from build123d import *

# Parameters (mm, degrees)
F0_W          = 1700
F0_H          = 290
F1_DEPTH      = 30
F2_W          = 30
F2_H          = 30
F3_DEPTH      = 600
F4_W          = 290
F4_H          = 30
F5_DEPTH      = 850
F5_DEPTH_BACK = 850


with BuildPart() as f1:
    # F0 (on Top) → F1 (new body)
    with BuildSketch(Plane.XY):
        Rectangle(F0_W, F0_H)
    extrude(amount=F1_DEPTH)

    # F2 (on face) → F3 (join)
    with BuildSketch(Plane(origin=(0, 0, 0), x_dir=(1, 0, 0), z_dir=(0, 0, -1))):
        with Locations((-835, 130)):
            Rectangle(F2_W, F2_H)
        with Locations((835, 130)):
            Rectangle(F2_W, F2_H)
        with Locations((835, -130)):
            Rectangle(F2_W, F2_H)
        with Locations((-835, -130)):
            Rectangle(F2_W, F2_H)
    extrude(amount=F3_DEPTH)

    # F4 (on Right) → F5 (join, two sides)
    with BuildSketch(Plane.YZ) as f5_sk:
        with Locations((0, -315)):
            Rectangle(F4_W, F4_H)
    extrude(amount=F5_DEPTH)
    extrude(f5_sk.sketch, amount=-F5_DEPTH_BACK)


solid = f1.part
Work out the finished part from the listing and answer in its coordinate system (mm). A direction names the side the tool comes from. Coordinates: 2 decimals unless noted, no trailing zeros. Write each loop counter-clockwise with the first axis right and the second up, starting at its lowest first coordinate (ties: lowest second). Pieces come first, ordered by that corner, then holes. Notation, with made-up numbers: M 22,-1 L 42,-1 A24 cw 42,33 Z; hole C 83.5,81.25 d8. An arc over 180 degrees is marked long. Use one line per item in the form item = value. Start each with the question number.
1. This flat-tipped pin is pushed along its axis until it touches: P1, Ø2, axis at x = -123, y = 34, coming from the -Z side. Where does it stop, or does it pass through?
2. Straight lines are drawn through the part: probe 1 along Z at (x, y) = (625.5, -29.5); probe 2 along X at (y, z) = (116.5, -101). For each, find the intervals that lie inside material, in ascending order. Write a range as from..to.
3. The part is cut by section C-C (y = -61). Give the vertices of the cut face in (x, z), plus the area to 3 significant figures.
4. The part is cut by section B-B (x = -293.5). Give the vertices of the cut face in (y, z).
5. A tool of negligible diameter and unlimited length cuts with its end or side. For faces 5 (the face through (820, 130, -148)), 6 (the face through (-835, -115, -148)), 7 (the face through (820, 130, -463)), from which of +Z, -Z, +X, -X, +Y, -Y can it reach the whole face along a straight path? Write none if from no direction.
6. The mould has two halves that part along Z. Classify faces 1 (the face through (835, 115, -463)), 2 (the face through (835, -130, -600)), 3 (the face through (835, 115, -148)), 4 (the face through (12, -2, -300)): released by +Z, released by -Z, zero draft, split by the parting line, or undercut.
7. The part is cut by section A-A (z = -104). Give the vertices of the cut face in (x, y).
Evaluation:
q1.P1 = -330
q2.probe_1 = -330..-300, 0..30
q2.probe_2 = -850..-820, 820..850
q3.outline = M -850,-330 L 850,-330 L 850,-300 L -850,-300 Z; M -850,0 L 850,0 L 850,30 L -850,30 Z
q3.area = 102,000 mm^2
q4.outline = M -145,-330 L 145,-330 L 145,-300 L -145,-300 Z; M -145,0 L 145,0 L 145,30 L -145,30 Z
q5.face_5 = +Y, -Y
q5.face_6 = +X, -X
q5.face_7 = -Z, +Y, -Y
q6.face_1 = zero draft
q6.face_2 = released by -Z
q6.face_3 = undercut
q6.face_4 = undercut
q7.outline = M -850,-145 L -820,-145 L -820,-115 L -850,-115 Z; M -850,115 L -820,115 L -820,145 L -850,145 Z; M 820,-145 L 850,-145 L 850,-115 L 820,-115 Z; M 820,115 L 850,115 L 850,145 L 820,145 Z
